Build history of the part. All positions in model axes, mm. A direction names the side the tool comes from. Give positions to 0.01 mm unless a question says otherwise; leave off trailing zeros. Order: outer loops, then holes, each group sorted by start corner. A loop starts at its lowest first (then second) coordinate and runs counter-clockwise, first axis right, second up. Notation, with made-up numbers: (83.25, 56.5) - (95.25, 56.5) arc R30 ccw to (95.25, 89.5) - close; hole circle Ø2 at (-0.5, -17). An arc over 180 degrees is marked (long way). One line per item, written item: value.
```python
from build123d import *

# Parameters (mm, degrees)
SKETCH1_R           = 2.95
BOSS_EXTRUDE1_DEPTH = 1
SKETCH5_R           = 0.3
BOSS_EXTRUDE2_DEPTH = 5


with BuildPart() as part:
    # Sketch1 → Boss-Extrude1 (new body)
    with BuildSketch(Plane(origin=(0, 0, 0), x_dir=(1, 0, 0), z_dir=(0, 1, 0))):
        with Locations(Location((0, 0, 0), (0, 0, 270))):
            Circle(SKETCH1_R)
    extrude(amount=BOSS_EXTRUDE1_DEPTH)

    # Sketch3 → Revolve1 (revolve)
    with BuildSketch(Plane.XY, mode=Mode.PRIVATE) as revolve1_sk:
        with BuildLine():
            Line((0, 1), (2.5, 1))
            Line((2.5, 1), (2.5, 6.5))
            ThreePointArc((2.5, 6.5), (1.767766953, 8.267766953), (0, 9))
            Line((0, 9), (0, 6.5))
            Line((0, 6.5), (0, 1))
        make_face()
    revolve(revolve1_sk.sketch.rotate(Axis((0, 1, 0), (0, 1, 0)), 90), axis=Axis((0, 1, 0), (0, 1, 0)))

    # Sketch5 → Boss-Extrude2 (add)
    with BuildSketch(Plane.XZ):
        with Locations(Location((0, 1.5, 0), (0, 0, 90))):
            Circle(SKETCH5_R)
    boss_extrude2 = extrude(amount=BOSS_EXTRUDE2_DEPTH)

    # Mirror1: Boss-Extrude2 across plane
    add(boss_extrude2.mirror(Plane.XY))


solid = part.part
```
(1) 3-axis set-ups, long thin cutter, end or side, ignore diameter. For faces 1 (the face through (-2.88, 0.49, -0.64)), 2 (the face through (-0.1, 3.8, 2.5)): which of +Z, -Z, +X, -X, +Y, -Y reach the whole face in a straight line?
Completed:
face 1: +Y, -Y
face 2: +Y
(2) Slice it at D-D, the plane x = 1.9. Give the cut face in (y, z).
Completed:
outline: (0, -2.26) - (1, -2.26) - (1, -1.62) - (6.5, -1.62) arc R1.62 ccw to (6.5, 1.62) - (1, 1.62) - (1, 2.26) - (0, 2.26) - close
(3) Slice it at B-B, the plane x = 0. Give the cut face in (y, z), and give its area (3 significant figures).
Completed:
outline: (-5, -1.8) - (0, -1.8) - (0, -2.95) - (1, -2.95) - (1, -2.5) - (6.5, -2.5) arc R2.5 ccw to (6.5, 2.5) - (1, 2.5) - (1, 2.95) - (0, 2.95) - (0, 1.8) - (-5, 1.8) - (-5, 1.2) - (0, 1.2) - (0, -1.2) - (-5, -1.2) - close
area: 49.2 mm²
(4) Pin check, flat tips, straight feed: P1, Ø1.5, axis at x = -2, z = 1.5, coming from the -Y side; P2, Ø2, axis at y = 1.5, z = 2, coming from the +X side. Stop position of each tip, or through.
Completed:
P1: y = 0
P2: x = 2.72
(5) Slice it at C-C, the plane y = 4.5. Give the cut face in (x, z), and give its area (3 significant figures).
Completed:
outline: circle Ø5 at (0, 0)
area: 19.6 mm²
(6) Drill centre lines: line 1 (Y direction, x = 1.4, z = -2.35); line 2 (Z direction, x = -1.75, y = 1.5); line 3 (Z direction, x = 2.3, y = 4). Where is each one in solid material? Low to high.
Completed:
line 1: 0 to 1
line 2: -1.79 to 1.79
line 3: -0.98 to 0.98
(7) Slice it at A-A, the plane z = 0. Give the cut face in (x, y), and give its area (3 significant figures).
Completed:
outline: (-2.95, 0) - (2.95, 0) - (2.95, 1) - (2.5, 1) - (2.5, 6.5) arc R2.5 ccw to (-2.5, 6.5) - (-2.5, 1) - (-2.95, 1) - close
area: 43.2 mm²
